from build123d import *

# Parameters (mm, degrees)
SKETCH1_W             = 203.2
SKETCH1_H             = 368.3
BOSS_EXTRUDE4_DEPTH   = 254
BOSS_EXTRUDE4_TAPER   = 11.25
CUT_EXTRUDE1_DEPTH    = 254
BOSS_EXTRUDE5_START   = -151.75
BOSS_EXTRUDE5_DEPTH   = 102
BODY_MOVE_COPY1_ANGLE = 180


with BuildPart() as part:
    # Sketch1 → Boss-Extrude4 (new body)
    with BuildSketch(Plane(origin=(0, 0, 0), x_dir=(1, 0, 0), z_dir=(0, 1, 0))):
        with Locations((-183.252356021, -50.101832461)):
            Rectangle(SKETCH1_W, SKETCH1_H)
    extrude(amount=BOSS_EXTRUDE4_DEPTH, taper=BOSS_EXTRUDE4_TAPER)

    # Sketch2 → Cut-Extrude1 (cut)
    with BuildSketch(Plane(origin=(-82.7176, 0, 0), x_dir=(0, 0, -1), z_dir=(1, 0, 0))):
        Polygon((-234.106807468, 0), (147.485457697, 0), (93.149429588, 234.95), (-191.90501696, 215.9), align=None)
    extrude(amount=-CUT_EXTRUDE1_DEPTH, mode=Mode.SUBTRACT)


with BuildPart() as cut_extrude1_kept_piece:
    # of the separate pieces the step leaves, the one the design keeps (cut_extrude1_pieces_kept)
    add(part.part.solids().sort_by_distance((-238.194452935, 234.565118806, -87.390264453))[0])

    # Sketch3 → Boss-Extrude5 (add)
    with BuildSketch(Plane(origin=(-82.7176, 0, 0), x_dir=(0, 0, -1), z_dir=(1, 0, 0)).offset(BOSS_EXTRUDE5_START)):
        Polygon((-183.728091146, 254), (-231.967371745, 254), (-231.967371745, 234.95), (-187.517371745, 234.95), align=None)
    extrude(amount=BOSS_EXTRUDE5_DEPTH)


with BuildPart() as cut_extrude1_kept_piece_1:
    # Body-Move/Copy1: moved
    add(cut_extrude1_kept_piece.part.rotate(Axis((-183.252356021, 234.970263522, 0), (0, 0, 1)), BODY_MOVE_COPY1_ANGLE))


solid = cut_extrude1_kept_piece_1.part
For this review, take the finished solid that the model builds, in its own axes (mm). Give positions to 0.01 mm unless a question says otherwise; leave off trailing zeros. One line per question, with ' | ' between items.
1) Insertion check: pin 1 Ø8 at (x, z) = (-202.5, 73.5) entering from +Y; pin 2 Ø8 at (x, z) = (-209.5, 136.5) entering from +Y; pin 3 Ø9.5 at (y, z) = (227.5, 207) entering from +X. Each pin has a flat end and moves straight along its axis. Give the tip position at first contact, or say it passes through.
Resolved:
pin 1: stops at y = 246.39 | pin 2: stops at y = 250.61 | pin 3: stops at x = -132.04
2) To check wall thickness, follow probe 1 along Y at (x, z) = (-230, 207.5); probe 2 along Y at (x, z) = (-146.5, 25.5); probe 3 along Z at (x, y) = (-166.5, 227). State the ranges of each line that lie inside material, in increasing order.
Resolved:
probe 1: y = 215.94 to 234.99 | probe 2: y = 215.94 to 242.92 | probe 3: z = -85.72 to 231.97
3) The part is to be moulded in two halves that separate along Y. For faces 1 (the flat face through (-182, 215.941, 72)), 2 (the flat face through (-234.037, 225, 208)), 3 (the flat face through (-184.073, 244.557, 50.003)), say which applies: +Y half, -Y half, draft (parallel to the pull), parting line (faces both ways), or undercut.
Resolved:
face 1: -Y half | face 2: draft | face 3: +Y half
